```python
from build123d import *

# Parameters (mm, degrees)
EXTRUDE_1_DEPTH = 3
SKETCH_2_R      = 0.6
SKETCH_2_R_2    = 1.25
EXTRUDE_2_DEPTH = 2
SKETCH_3_R      = 5.5
EXTRUDE_3_DEPTH = 2
SKETCH_4_R      = 5.5
EXTRUDE_5_DEPTH = 4


# Read off the part's stored shape, not the designer's step: 填料-伸長1
with BuildPart() as part:
    # 填料-伸長1 outline → 填料-伸長1 (new body)
    with BuildSketch(Plane(origin=(0, 14.156954032, 0), x_dir=(1, 0, 0), z_dir=(0, 1, 0))):
        with BuildLine():
            Line((-82.339013046, -221.365982672), (-68.587342058, -223.095847576))
            ThreePointArc((-68.587342058, -223.095847576), (-65.812443105, -224.067756352), (-62.933383432, -223.471361963))
            Line((-62.933383432, -223.471361963), (-49.073726982, -223.575336213))
            ThreePointArc((-49.073726982, -223.575336213), (-44.993021918, -219.938385769), (-48.556901099, -215.793711169))
            Line((-48.556901099, -215.793711169), (-62.308572088, -214.063846266))
            ThreePointArc((-62.308572088, -214.063846266), (-65.08347104, -213.091937489), (-67.962530713, -213.688331878))
            Line((-67.962530713, -213.688331878), (-81.822187163, -213.584357628))
            ThreePointArc((-81.822187163, -213.584357628), (-85.902892228, -217.221308072), (-82.339013046, -221.365982672))
        make_face()
        with BuildLine():
            Line((-49.024567087, -221.975659985), (-63.351091856, -221.868183318))
            ThreePointArc((-63.351091856, -221.868183318), (-65.706410804, -222.471273609), (-67.96128377, -221.561991939))
            Line((-67.96128377, -221.561991939), (-82.176185543, -219.773855813))
            ThreePointArc((-82.176185543, -219.773855813), (-84.306409484, -217.327340372), (-81.871347058, -215.184033856))
            Line((-81.871347058, -215.184033856), (-67.544822289, -215.291510523))
            ThreePointArc((-67.544822289, -215.291510523), (-65.189503341, -214.688420233), (-62.934630375, -215.597701902))
            Line((-62.934630375, -215.597701902), (-48.719728602, -217.385838028))
            ThreePointArc((-48.719728602, -217.385838028), (-46.589504661, -219.832353469), (-49.024567087, -221.975659985))
        make_face(mode=Mode.SUBTRACT)
    extrude(amount=EXTRUDE_1_DEPTH)

    # 草圖2 → 填料-伸長2 (add)
    with BuildSketch(Plane(origin=(0, 17.156954032, 0), x_dir=(1, 0, 0), z_dir=(0, 1, 0))):
        with BuildLine():
            Line((-82.339013046, -221.365982672), (-68.587342058, -223.095847576))
            ThreePointArc((-68.587342058, -223.095847576), (-65.812443105, -224.067756352), (-62.933383432, -223.471361963))
            Line((-62.933383432, -223.471361963), (-49.073726982, -223.575336213))
            ThreePointArc((-49.073726982, -223.575336213), (-44.993021918, -219.938385769), (-48.556901099, -215.793711169))
            Line((-48.556901099, -215.793711169), (-62.308572088, -214.063846266))
            ThreePointArc((-62.308572088, -214.063846266), (-65.08347104, -213.091937489), (-67.962530713, -213.688331878))
            Line((-67.962530713, -213.688331878), (-81.822187163, -213.584357628))
            ThreePointArc((-81.822187163, -213.584357628), (-85.902892228, -217.221308072), (-82.339013046, -221.365982672))
        make_face()
        with Locations(Location((-48.185987405, -219.726321168, 0), (0, 0, 270))):
            Circle(SKETCH_2_R, mode=Mode.SUBTRACT)
        with Locations(Location((-50.281371006, -219.587153774, 0), (0, 0, 270))):
            Circle(SKETCH_2_R, mode=Mode.SUBTRACT)
        with Locations(Location((-52.376754608, -219.44798638, 0), (0, 0, 270))):
            Circle(SKETCH_2_R, mode=Mode.SUBTRACT)
        with Locations(Location((-54.472138209, -219.308818985, 0), (0, 0, 270))):
            Circle(SKETCH_2_R, mode=Mode.SUBTRACT)
        with Locations(Location((-56.56752181, -219.169651591, 0), (0, 0, 270))):
            Circle(SKETCH_2_R, mode=Mode.SUBTRACT)
        with Locations(Location((-58.662905411, -219.030484197, 0), (0, 0, 270))):
            Circle(SKETCH_2_R, mode=Mode.SUBTRACT)
        with Locations(Location((-65.447957073, -218.579846921, 0), (0, 0, 270))):
            Circle(SKETCH_2_R_2, mode=Mode.SUBTRACT)
        with Locations(Location((-72.233008734, -218.129209644, 0), (0, 0, 270))):
            Circle(SKETCH_2_R, mode=Mode.SUBTRACT)
        with Locations(Location((-74.328392335, -217.99004225, 0), (0, 0, 270))):
            Circle(SKETCH_2_R, mode=Mode.SUBTRACT)
        with Locations(Location((-76.423775936, -217.850874856, 0), (0, 0, 270))):
            Circle(SKETCH_2_R, mode=Mode.SUBTRACT)
        with Locations(Location((-78.519159538, -217.711707461, 0), (0, 0, 270))):
            Circle(SKETCH_2_R, mode=Mode.SUBTRACT)
        with Locations(Location((-80.614543139, -217.572540067, 0), (0, 0, 270))):
            Circle(SKETCH_2_R, mode=Mode.SUBTRACT)
        with Locations(Location((-82.70992674, -217.433372673, 0), (0, 0, 270))):
            Circle(SKETCH_2_R, mode=Mode.SUBTRACT)
    extrude(amount=EXTRUDE_2_DEPTH)

    # 草圖3 → 填料-伸長3 (add)
    with BuildSketch(Plane(origin=(0, 19.156954032, 0), x_dir=(1, 0, 0), z_dir=(0, 1, 0))):
        with Locations(Location((-65.447957073, -218.579846921, 0), (0, 0, 117.206266925))):
            Circle(SKETCH_3_R)
    extrude(amount=EXTRUDE_3_DEPTH)

    # 草圖4 → 填料-伸長5 (add)
    with BuildSketch(Plane(origin=(0, 21.156954032, 0), x_dir=(1, 0, 0), z_dir=(0, 1, 0))):
        with BuildLine():
            Line((-65.841884706, -181.758677002), (-67.962530713, -213.688331878))
            ThreePointArc((-67.962530713, -213.688331878), (-66.686272082, -213.221061989), (-65.334397341, -213.081019392))
            Line((-65.334397341, -213.081019392), (-63.345192567, -183.146990755))
            Line((-63.345192567, -183.146990755), (-62.84629171, -183.180125849))
            Line((-62.84629171, -183.180125849), (-64.834397341, -213.114177295))
            ThreePointArc((-64.834397341, -213.114177295), (-63.512339264, -213.431703207), (-62.308572088, -214.063846266))
            Line((-62.308572088, -214.063846266), (-60.187926081, -182.134191389))
            Line((-60.187926081, -182.134191389), (-65.841884706, -181.758677002))
        make_face()
        with BuildLine():
            Line((-28.626787154, -218.185919287), (-60.55644203, -216.06527328))
            ThreePointArc((-60.55644203, -216.06527328), (-60.102242306, -217.286272944), (-59.947957073, -218.579846921))
            ThreePointArc((-59.947957073, -218.579846921), (-59.94806161, -218.613757162), (-59.94837522, -218.647666115))
            Line((-59.94837522, -218.647666115), (-30.05766404, -220.633992316))
            Line((-30.05766404, -220.633992316), (-30.090799133, -221.132893173))
            Line((-30.090799133, -221.132893173), (-59.977374886, -219.147940697))
            ThreePointArc((-59.977374886, -219.147940697), (-60.291810853, -220.494045491), (-60.931956418, -221.719231906))
            Line((-60.931956418, -221.719231906), (-29.002301541, -223.839877913))
            Line((-29.002301541, -223.839877913), (-28.626787154, -218.185919287))
        make_face()
        with Locations(Location((-65.447957073, -218.579846921, 0), (0, 0, 117.206266925))):
            Circle(SKETCH_4_R)
        with BuildLine():
            ThreePointArc((-66.061516804, -224.045516546), (-67.383574881, -223.727990635), (-68.587342058, -223.095847576))
            Line((-68.587342058, -223.095847576), (-70.707988065, -255.025502452))
            Line((-70.707988065, -255.025502452), (-65.054029439, -255.401016839))
            Line((-65.054029439, -255.401016839), (-62.933383432, -223.471361963))
            ThreePointArc((-62.933383432, -223.471361963), (-64.209643695, -223.938632229), (-65.561520152, -224.07867438))
            Line((-65.561520152, -224.07867438), (-67.544665601, -253.921520844))
            Line((-67.544665601, -253.921520844), (-68.043566458, -253.88838575))
            Line((-68.043566458, -253.88838575), (-66.061516804, -224.045516546))
        make_face()
        with BuildLine():
            ThreePointArc((-70.908334203, -217.920846468), (-70.588006225, -216.622835241), (-69.963957728, -215.440461936))
            Line((-69.963957728, -215.440461936), (-101.893612604, -213.319815929))
            Line((-101.893612604, -213.319815929), (-102.269126991, -218.973774554))
            Line((-102.269126991, -218.973774554), (-70.339472115, -221.094420561))
            ThreePointArc((-70.339472115, -221.094420561), (-70.811844008, -219.795871979), (-70.945650262, -218.420568553))
            Line((-70.945650262, -218.420568553), (-100.832194129, -216.434519282))
            Line((-100.832194129, -216.434519282), (-100.799059035, -215.935618425))
            Line((-100.799059035, -215.935618425), (-70.908334203, -217.920846468))
        make_face()
    extrude(amount=EXTRUDE_5_DEPTH)


solid = part.part
```
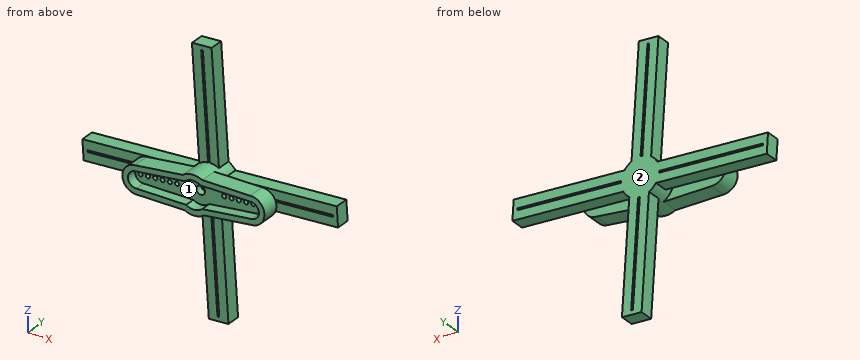
Verification items for the finished model (mm, model axes). Face numbers are marked on the shaded views. Coordinates: 2 decimals unless noted, no trailing zeros. Loops run counter-clockwise (first coordinate to the right, second up) from the corner with the lowest first, then second, coordinate; pieces in that order, holes last. Notation, with made-up numbers: (81, 25.5) -> (132, 25.5) arc R17 cw to (132, 41.5) -> close; hole circle Ø7 at (54.25, -33.5). An arc over 180 degrees is marked (long way). Answer in a Markdown table with one row per item.
1) Scan lines: line 1 along X through (y, z) = (21.25, 226.5); line 2 along Y through (x, z) = (-41.5, 217.5); line 3 along Z through (x, y) = (-83, 22.75). Record each from-to range of solid material in increasing order. Write a range as from..to.
The answers:
| item | result |
|---|---|
| line 1 | x = -68.81..-66.22, -65.72..-63.13 |
| line 2 | y = 21.16..25.16 |
| line 3 | z = 214.57..217.12, 217.62..220.25 |
2) Section check B-B (x = -37). Record the cut outline in (y, z).
The answers:
| item | result |
|---|---|
| outline | (21.16, 217.63) -> (25.16, 217.63) -> (25.16, 220.17) -> (21.16, 220.17) -> close; (21.16, 220.67) -> (25.16, 220.67) -> (25.16, 223.31) -> (21.16, 223.31) -> close |
3) Section check D-D (y = 22.5). Give the number of separate pieces and of enclosed holes in the cut face, and give its area (3 significant figures).
The answers:
| item | result |
|---|---|
| separate pieces | 1 |
| enclosed holes | 4 |
| area | 748 mm2 |
4) Draft check along X on the marked faces 1 and 2. Enter one of: released by +X, released by -X, zero draft, split by the parting line, or undercut.
The answers:
| item | result |
|---|---|
| face 1 | undercut |
| face 2 | zero draft |
5) Section check C-C (z = 229). Record the cut outline in (x, y), and give its area (3 significant figures).
The answers:
| item | result |
|---|---|
| outline | (-68.98, 21.16) -> (-66.39, 21.16) -> (-66.39, 25.16) -> (-68.98, 25.16) -> close; (-65.89, 21.16) -> (-63.3, 21.16) -> (-63.3, 25.16) -> (-65.89, 25.16) -> close |
| area | 20.7 mm2 |
6) Section check A-A (y = 15). Record the cut outline in (x, z).
The answers:
| item | result |
|---|---|
| outline | (-82.34, 221.37) arc R3.9 ccw to (-81.82, 213.58) -> (-67.96, 213.69) arc R5.5 ccw to (-62.31, 214.06) -> (-48.56, 215.79) arc R3.9 ccw to (-49.07, 223.58) -> (-62.93, 223.47) arc R5.5 ccw to (-68.59, 223.1) -> close; hole (-82.18, 219.77) arc R2.3 ccw to (-81.87, 215.18) -> (-67.54, 215.29) arc R3.9 ccw to (-62.93, 215.6) -> (-48.72, 217.39) arc R2.3 ccw to (-49.02, 221.98) -> (-63.35, 221.87) arc R3.9 ccw to (-67.96, 221.56) -> close |
7) Depth check by flat-ended pin: P1, Ø1.4, axis at x = -76.42, z = 217.85, coming from the +Y side; P2, Ø1.5, axis at x = -65.5, y = 18.5, coming from the -Z side; P3, Ø1.1, axis at x = -74.33, z = 217.99, coming from the -Y side; P4, Ø1.6, axis at x = -58.66, z = 219.03, coming from the -Y side. Enter the tip coordinate at first touch or a pass-through.
The answers:
| item | result |
|---|---|
| P1 | stops at y = 25.16 |
| P2 | stops at z = 213.08 |
| P3 | stops at y = 21.16 |
| P4 | stops at y = 17.16 |
